```python
from build123d import *

# Parameters (mm, degrees)
SKETCH1_W           = 45
SKETCH1_H           = 45
BOSS_EXTRUDE1_DEPTH = 50
SKETCH4_R           = 15
BOSS_EXTRUDE2_DEPTH = 71
FILLET1_R           = 2
FILLET2_R           = 5
SKETCH5_R           = 2.5
BOSS_EXTRUDE3_DEPTH = 10
BOSS_EXTRUDE4_START = 10
SKETCH6_R           = 2.5
BOSS_EXTRUDE4_DEPTH = 10


with BuildPart() as part:
    # Sketch1 → Boss-Extrude1 (new body)
    with BuildSketch(Plane.XY):
        Rectangle(SKETCH1_W, SKETCH1_H)
    extrude(amount=BOSS_EXTRUDE1_DEPTH)

    # Sketch4 → Boss-Extrude2 (add)
    with BuildSketch(Plane.XZ.offset(22.5)):
        with Locations(Location((0, 25, 0), (0, 0, 270))):
            Circle(SKETCH4_R)
    extrude(amount=BOSS_EXTRUDE2_DEPTH)

    # Fillet1
    fillet1_edges = [part.edges().sort_by_distance(p)[0] for p in [
        (-22.5, 0, 50),
        (22.5, 0, 50),
        (22.5, -22.5, 25),
        (-22.5, -22.5, 25),
        (-22.5, 22.5, 25),
        (22.5, 22.5, 25),
    ]]
    fillet(fillet1_edges, radius=FILLET1_R)

    # Fillet2
    fillet2_edges = [part.edges().sort_by_distance(p)[0] for p in [
        (0, -22.5, 40),
    ]]
    fillet(fillet2_edges, radius=FILLET2_R)

    # Sketch5 → Boss-Extrude3 (add)
    with BuildSketch(Plane.XY.offset(50)):
        Circle(SKETCH5_R)
    extrude(amount=BOSS_EXTRUDE3_DEPTH)

    # Sketch6 → Boss-Extrude4 (add)
    with BuildSketch(Plane(origin=(0, 0, 0), x_dir=(-1, 0, 0), z_dir=(0, 0, -1)).offset(BOSS_EXTRUDE4_START)):
        with Locations(Location((0, 0, 0), (0, 0, 180))):
            Circle(SKETCH6_R)
    extrude(amount=-BOSS_EXTRUDE4_DEPTH)


solid = part.part
```
Build history of the part. All positions in model axes, mm. A direction names the side the tool comes from. Coordinates: 2 decimals unless noted, no trailing zeros. Order: outer loops, then holes, each group sorted by start corner. A loop starts at its lowest first (then second) coordinate and runs counter-clockwise, first axis right, second up.
Item 1: Saw through at A-A on x = 0. List the corners of the cut face in (y, z).
Filled in:
outline: (-93.5, 10) - (-27.5, 10) arc R5 cw to (-22.5, 5) - (-22.5, 0) - (-2.5, 0) - (-2.5, -10) - (2.5, -10) - (2.5, 0) - (22.5, 0) - (22.5, 50) - (2.5, 50) - (2.5, 60) - (-2.5, 60) - (-2.5, 50) - (-22.5, 50) - (-22.5, 45) arc R5 cw to (-27.5, 40) - (-93.5, 40) - close
Item 2: Saw through at B-B on y = 0. List the corners of the cut face in (x, z).
Filled in:
outline: (-22.5, 0) - (-2.5, 0) - (-2.5, -10) - (2.5, -10) - (2.5, 0) - (22.5, 0) - (22.5, 48) arc R2 ccw to (20.5, 50) - (2.5, 50) - (2.5, 60) - (-2.5, 60) - (-2.5, 50) - (-20.5, 50) arc R2 ccw to (-22.5, 48) - close
Item 3: Tool access for faces 1 (the flat face through (22.5, 0, 24)), 2 (the cylindrical face through (-2.5, -0.1, -5.1)), 3 (the flat face through (-19, -22.5, 14)), 4 (the flat face through (0, 0, 60)), 5 (the cylindrical face through (-0.54, -2.44, 54.93)): list every direction of +Z, -Z, +X, -X, +Y, -Y with a clear straight run to the whole face (end or side of a thin tool).
Filled in:
face 1: +Z, -Z, +X, +Y, -Y
face 2: -Z
face 3: -Y
face 4: +Z, +X, -X, +Y, -Y
face 5: +Z
Item 4: Saw through at D-D on y = 13.5. List the corners of the cut face in (x, z).
Filled in:
outline: (-22.5, 0) - (22.5, 0) - (22.5, 48) arc R2 ccw to (20.5, 50) - (-20.5, 50) arc R2 ccw to (-22.5, 48) - close
Item 5: Saw through at C-C on z = 25. List the corners of the cut face in (x, y).
Filled in:
outline: (-22.5, -20.5) arc R2 ccw to (-20.5, -22.5) - (-20, -22.5) arc R5 cw to (-15, -27.5) - (-15, -93.5) - (15, -93.5) - (15, -27.5) arc R5 cw to (20, -22.5) - (20.5, -22.5) arc R2 ccw to (22.5, -20.5) - (22.5, 20.5) arc R2 ccw to (20.5, 22.5) - (-20.5, 22.5) arc R2 ccw to (-22.5, 20.5) - close
Item 6: Drill centre lines: L1, parallel to Y at x = 19.5, z = 10.5; L2, parallel to Z at x = 16.5, y = -5.5; L3, parallel to Y at x = -16, z = 25. Where is each one in solid material? Low to high.
Filled in:
L1: y = -22.5 to 22.5
L2: z = 0 to 50
L3: y = -24.5 to 22.5
Item 7: Drop flat-ended pins along their axis: pin 1 Ø8 at (x, y) = (-4, -73.5) entering from -Z; pin 2 Ø3 at (y, z) = (-56.5, 40) entering from -X; pin 3 Ø13.5 at (x, y) = (10, 10) entering from -Z. Give the stop position or say it passes through.
Filled in:
pin 1: stops at z = 10
pin 2: stops at x = -6.54
pin 3: stops at z = 0
